from build123d import *

# Parameters (mm, degrees)
SKETCH_1_R               = 1.65
SKETCH_1_R_2             = 1.25
EXTRUDE_4_DEPTH          = 3
SKETCH_4_W               = 52
SKETCH_4_H               = 3
EXTRUDE_6_DEPTH          = 16
CUT_EXTRUDE_1_DEPTH      = 81.034703796
CUT_EXTRUDE_1_DEPTH_BACK = 22
SKETCH_3_R               = 1.65
FILLET_1_R               = 2


with BuildPart() as part:
    # 草图1 → 凸台-拉伸4 (new body)
    with BuildSketch(Plane(origin=(0, 0, 0), x_dir=(0, 0, -1), z_dir=(1, 0, 0))):
        with BuildLine():
            Line((61, 13), (52.5, 53))
            Line((52.5, 53), (23.619851789, 62.203688194))
            ThreePointArc((23.619851789, 62.203688194), (4.878186687, 58.71413126), (-2.572313303, 41.16656538))
            Line((-2.572313303, 41.16656538), (0, 13))
            Line((0, 13), (61, 13))
        make_face()
        with BuildLine():
            Line((28.220139039, 48.391717332), (29.643651042, 47.578281902))
            ThreePointArc((29.643651042, 47.578281902), (32.668112531, 47.193796374), (30.257622978, 45.32705147))
            Line((30.257622978, 45.32705147), (29.463156964, 43.936735946))
            ThreePointArc((29.463156964, 43.936735946), (27.918719173, 37.045985315), (22.766171662, 32.217011666))
            Line((22.766171662, 32.217011666), (21.972102707, 30.827390996))
            ThreePointArc((21.972102707, 30.827390996), (21.587617178, 27.802929507), (19.720872274, 30.21341906))
            Line((19.720872274, 30.21341906), (18.298407802, 31.026255901))
            ThreePointArc((18.298407802, 31.026255901), (11.546134207, 32.58073487), (6.778813424, 37.60888126))
            Line((6.778813424, 37.60888126), (5.221211801, 38.49893933))
            ThreePointArc((5.221211801, 38.49893933), (2.196750311, 38.883424859), (4.607239865, 40.750169763))
            Line((4.607239865, 40.750169763), (5.51775044, 42.34356327))
            ThreePointArc((5.51775044, 42.34356327), (7.080883762, 48.953319836), (11.981852501, 53.655741877))
            Line((11.981852501, 53.655741877), (12.892760135, 55.249830237))
            ThreePointArc((12.892760135, 55.249830237), (13.277245664, 58.274291726), (15.143990568, 55.863802173))
            Line((15.143990568, 55.863802173), (16.702639721, 54.973145514))
            ThreePointArc((16.702639721, 54.973145514), (23.453468727, 53.418570281), (28.220139039, 48.391717332))
        make_face(mode=Mode.SUBTRACT)
        with Locations((48.441115069, 36.836873887)):
            Circle(SKETCH_1_R, mode=Mode.SUBTRACT)
        with Locations((38.518336301, 19.472011044)):
            Circle(SKETCH_1_R, mode=Mode.SUBTRACT)
        with Locations((53.026104064, 18.242284788)):
            Circle(SKETCH_1_R, mode=Mode.SUBTRACT)
        with Locations((48.125, 48)):
            Circle(SKETCH_1_R, mode=Mode.SUBTRACT)
        with Locations((3.788610616, 19.472011044)):
            Circle(SKETCH_1_R, mode=Mode.SUBTRACT)
        with Locations((23.354935737, 21.197394906)):
            Circle(SKETCH_1_R_2, mode=Mode.SUBTRACT)
    extrude(amount=EXTRUDE_4_DEPTH)

    # 草图4 → 凸台-拉伸6 (add)
    with BuildSketch(Plane(origin=(3, 0, 0), x_dir=(0, 0, -1), z_dir=(1, 0, 0))):
        with Locations((35, 11.5)):
            Rectangle(SKETCH_4_W, SKETCH_4_H)
    extrude(amount=-EXTRUDE_6_DEPTH)

    # 草图3 → 切除-拉伸1 (cut, two sides: drawn at the far end of the back side and taken through both)
    with BuildSketch(Plane(origin=(0, 13, 0), x_dir=(1, 0, 0), z_dir=(0, 1, 0)).offset(-CUT_EXTRUDE_1_DEPTH_BACK)):
        with Locations(Location((-8.6, 56.35, 0), (0, 0, 90))):
            Circle(SKETCH_3_R)
        with Locations(Location((-8.6, 47.65, 0), (0, 0, 90))):
            Circle(SKETCH_3_R)
        with Locations(Location((-8.6, 22.3, 0), (0, 0, 90))):
            Circle(SKETCH_3_R)
        with Locations(Location((-8.6, 13.6, 0), (0, 0, 90))):
            Circle(SKETCH_3_R)
    extrude(amount=CUT_EXTRUDE_1_DEPTH + CUT_EXTRUDE_1_DEPTH_BACK, mode=Mode.SUBTRACT)

    # 圆角1
    fillet_1_edges = [part.edges().sort_by_distance(p)[0] for p in [
        (1.5, 13, 0),
        (-13, 11.5, -9),
        (-13, 11.5, -61),
        (1.5, 53, -52.5),
    ]]
    fillet(fillet_1_edges, radius=FILLET_1_R)


solid = part.part
Verification items for the finished model (mm, model axes). A direction names the side the tool comes from. Coordinates: 2 decimals unless noted, no trailing zeros. Order: outer loops, then holes, each group sorted by start corner. A loop starts at its lowest first (then second) coordinate and runs counter-clockwise, first axis right, second up.
1. Go/stop test with flat-tipped pins: pin 1 Ø3 at (y, z) = (49, -26) entering from -X; pin 2 Ø25 at (y, z) = (38.5, -19) entering from -X; pin 3 Ø4 at (x, z) = (-3.5, -23.5) entering from +Y; pin 4 Ø1.5 at (x, y) = (-7, 11.5) entering from +Z. Record where each tip stops, or that it passes through.
Results found:
pin 1: passes through
pin 2: stops at x = 0
pin 3: stops at y = 13
pin 4: stops at z = -9
2. Release check for a two-part mould opening along Z. For faces 1 (the face through (1.5, 20.7, -24.5)), 2 (the face through (-12.43, 11.52, -60.4)), 3 (the face through (-12.4, 11.52, -9.57)) record: +Z half, -Z half, draft (parallel to the pull), parting line (faces both ways), or undercut.
Results found:
face 1: undercut
face 2: -Z half
face 3: +Z half
3. Set-up check for faces 4 (the face through (-7, 11.5, -13.2)), 5 (the face through (1.479, 55.425, -15.912)), 6 (the face through (1, 13, -5)): record each of +Z, -Z, +X, -X, +Y, -Y from which the full face is reachable in a straight line by a thin tool's end or side.
Results found:
face 4: +Y, -Y
face 5: +X, -X
face 6: +Z, +X, -X, -Y
4. Scan lines: line 1 (X direction, y = 11.55, z = -56.35); line 2 (X direction, y = 41.5, z = -51.5); line 3 (Y direction, x = -11.5, z = -56). Record each from-to range of solid material in increasing order.
Results found:
line 1: x = -13 to -10.25, -6.95 to 3
line 2: x = 0 to 3
line 3: y = 10 to 13
5. Sectioned sample at A-A, the plane z = -47.65. Record the cut outline in (x, y).
Results found:
outline: (-13, 10) - (-10.25, 10) - (-10.25, 13) - (-13, 13) - close; (-6.95, 10) - (3, 10) - (3, 35.39) - (0, 35.39) - (0, 13) - (-6.95, 13) - close; (0, 38.28) - (3, 38.28) - (3, 46.42) - (0, 46.42) - close; (0, 49.58) - (3, 49.58) - (3, 54.55) - (0, 54.55) - close
6. Sectioned sample at D-D, the plane y = 34.5. Record the cut outline in (x, z).
Results found:
outline: (0, -56.43) - (3, -56.43) - (3, -25.97) - (0, -25.97) - close; (0, -9.03) - (3, -9.03) - (3, 1.96) - (0, 1.96) - close
7. Sectioned sample at B-B, the plane x = -7.75. Record the cut outline in (y, z).
Results found:
outline: (10, -61) - (13, -61) - (13, -57.76) - (10, -57.76) - close; (10, -54.94) - (13, -54.94) - (13, -49.06) - (10, -49.06) - close; (10, -46.24) - (13, -46.24) - (13, -23.71) - (10, -23.71) - close; (10, -20.89) - (13, -20.89) - (13, -15.01) - (10, -15.01) - close; (10, -12.19) - (13, -12.19) - (13, -9) - (10, -9) - close
8. Sectioned sample at C-C, the plane z = -56.35. Record the cut outline in (x, y).
Results found:
outline: (-13, 10) - (-10.25, 10) - (-10.25, 13) - (-13, 13) - close; (-6.95, 10) - (3, 10) - (3, 34.88) - (0, 34.88) - (0, 13) - (-6.95, 13) - close
